```python
from build123d import *

# Parameters (mm, degrees)
BOSS_EXTRUDE1_DEPTH     = 28.8
CUT_EXTRUDE1_DEPTH      = 41.90409515
BOSS_EXTRUDE3_DEPTH     = 1
CUT_EXTRUDE2_DEPTH      = 4.7
BOSS_EXTRUDE2_START     = -0.8
BOSS_EXTRUDE2_OUTLINE_R = 2.3
BOSS_EXTRUDE2_DEPTH     = 0.8
SKETCH5_OUTSIDE_W       = 57.418
SKETCH5_OUTSIDE_H       = 48.718
CUT_EXTRUDE3_DEPTH      = 3.5
SKETCH6_OUTSIDE_W       = 57.418
SKETCH6_OUTSIDE_H       = 48.718
CUT_EXTRUDE4_DEPTH      = 2.5
SKETCH8_W               = 6.84
SKETCH8_H               = 4.95
BOSS_EXTRUDE4_DEPTH     = 25


# Read off the part's stored shape, not the designer's step: Boss-Extrude2
with BuildPart() as part:
    # Sketch1 → Boss-Extrude1 (new body)
    with BuildSketch(Plane(origin=(0, 0, 0), x_dir=(1, 0, 0), z_dir=(0, 1, 0))):
        with BuildLine():
            Line((-4, 13.05), (4, 13.05))
            ThreePointArc((4, 13.05), (8.213640499, 11.465985784), (11.656602829, 8.566006872))
            ThreePointArc((11.656602829, 8.566006872), (12.685480206, 7.779523995), (13.95, 7.5))
            Line((13.95, 7.5), (25.95, 7.5))
            Line((25.95, 7.5), (25.95, -7.5))
            Line((25.95, -7.5), (13.95, -7.5))
            ThreePointArc((13.95, -7.5), (12.685480206, -7.779523995), (11.656602829, -8.566006872))
            ThreePointArc((11.656602829, -8.566006872), (8.213640499, -11.465985784), (4, -13.05))
            Line((4, -13.05), (-4, -13.05))
            ThreePointArc((-4, -13.05), (-17.05, 0), (-4, 13.05))
        make_face()
    extrude(amount=-BOSS_EXTRUDE1_DEPTH)

    # Sketch2 → Cut-Extrude1 (cut, through all)
    with BuildSketch(Plane(origin=(0, 0, 0), x_dir=(1, 0, 0), z_dir=(0, 1, 0))):
        with BuildLine():
            Line((0, -9.05), (-4.7, -9.05))
            ThreePointArc((-4.7, -9.05), (-13.75, 0), (-4.7, 9.05))
            Line((-4.7, 9.05), (0, 9.05))
            ThreePointArc((0, 9.05), (9.05, 0), (0, -9.05))
        make_face()
    extrude(amount=-CUT_EXTRUDE1_DEPTH, mode=Mode.SUBTRACT)

    # Sketch7 → Boss-Extrude3 (add)
    with BuildSketch(Plane(origin=(0, 0, 0), x_dir=(1, 0, 0), z_dir=(0, 1, 0))):
        with BuildLine():
            Line((-4.7, 10.05), (0, 10.05))
            ThreePointArc((0, 10.05), (10.05, 0), (0, -10.05))
            Line((0, -10.05), (-4.7, -10.05))
            ThreePointArc((-4.7, -10.05), (-14.75, 0), (-4.7, 10.05))
        make_face()
    extrude(amount=-BOSS_EXTRUDE3_DEPTH)

    # Sketch3 → Cut-Extrude2 (cut)
    with BuildSketch(Plane(origin=(0, 0, 0), x_dir=(1, 0, 0), z_dir=(0, 1, 0))):
        with BuildLine():
            Line((25.95, 7.5), (18.35, 7.5))
            ThreePointArc((18.35, 7.5), (19.55, 0), (18.35, -7.5))
            Line((18.35, -7.5), (25.95, -7.5))
            Line((25.95, -7.5), (25.95, 7.5))
        make_face()
    extrude(amount=-CUT_EXTRUDE2_DEPTH, mode=Mode.SUBTRACT)

    # Boss-Extrude2 outline → Boss-Extrude2 (add)
    # profile 1 of 2: a face of its own
    with BuildSketch(Plane(origin=(0, -15.8, 0), x_dir=(1, 0, 0), z_dir=(0, 1, 0)).offset(BOSS_EXTRUDE2_START)):
        with BuildLine():
            Line((17.95, -13.1), (17.95, -12.5))
            Line((17.95, -12.5), (18.65, -12.5))
            Line((18.65, -12.5), (18.65, -7.5))
            Line((18.65, -7.5), (13.95, -7.5))
            ThreePointArc((13.95, -7.5), (12.685480206, -7.779523995), (11.656602829, -8.566006872))
            ThreePointArc((11.656602829, -8.566006872), (9.898058886, -10.29612198), (7.85, -11.671341923))
            Line((7.85, -11.671341923), (7.85, -12.335141167))
            ThreePointArc((7.85, -12.335141167), (7.996446609, -12.688694558), (8.35, -12.835141167))
            Line((8.35, -12.835141167), (9.85, -12.835141167))
            Line((9.85, -12.835141167), (9.85, -13.1))
            ThreePointArc((9.85, -13.1), (13.9, -17.15), (17.95, -13.1))
        make_face()
        with Locations((13.9, -13.1)):
            Circle(BOSS_EXTRUDE2_OUTLINE_R, mode=Mode.SUBTRACT)
    # profile 2 of 2: a face of its own
    with BuildSketch(Plane(origin=(0, -15.8, 0), x_dir=(1, 0, 0), z_dir=(0, 1, 0)).offset(BOSS_EXTRUDE2_START)):
        with BuildLine():
            Line((17.95, 12.5), (17.95, 13.1))
            ThreePointArc((17.95, 13.1), (13.9, 17.15), (9.85, 13.1))
            Line((9.85, 13.1), (9.85, 12.835141167))
            Line((9.85, 12.835141167), (8.35, 12.835141167))
            ThreePointArc((8.35, 12.835141167), (7.996446609, 12.688694558), (7.85, 12.335141167))
            Line((7.85, 12.335141167), (7.85, 11.671341923))
            ThreePointArc((7.85, 11.671341923), (9.898058886, 10.29612198), (11.656602829, 8.566006872))
            ThreePointArc((11.656602829, 8.566006872), (12.685480206, 7.779523995), (13.95, 7.5))
            Line((13.95, 7.5), (18.65, 7.5))
            Line((18.65, 7.5), (18.65, 12.5))
            Line((18.65, 12.5), (17.95, 12.5))
        make_face()
        with Locations((13.9, 13.1)):
            Circle(BOSS_EXTRUDE2_OUTLINE_R, mode=Mode.SUBTRACT)
    extrude(amount=BOSS_EXTRUDE2_DEPTH)

    # Sketch5 outside → Cut-Extrude3 (cut)
    # profile 1 of 2: a face of its own
    with BuildSketch(Plane.XZ.offset(28.8)):
        with Locations((4.45, 0)):
            Rectangle(SKETCH5_OUTSIDE_W, SKETCH5_OUTSIDE_H)
        with BuildLine():
            Line((-4.7, -11.05), (0, -11.05))
            ThreePointArc((0, -11.05), (11.05, 0), (0, 11.05))
            Line((0, 11.05), (-4.7, 11.05))
            ThreePointArc((-4.7, 11.05), (-15.75, 0), (-4.7, -11.05))
        make_face(mode=Mode.SUBTRACT)
    # profile 2 of 2: a face of its own
    with BuildSketch(Plane.XZ.offset(28.8)):
        with BuildLine():
            Line((-4.7, 9.05), (0, 9.05))
            ThreePointArc((0, 9.05), (9.05, 0), (0, -9.05))
            Line((0, -9.05), (-4.7, -9.05))
            ThreePointArc((-4.7, -9.05), (-13.75, 0), (-4.7, 9.05))
        make_face()
    extrude(amount=-CUT_EXTRUDE3_DEPTH, mode=Mode.SUBTRACT)

    # Sketch6 outside → Cut-Extrude4 (cut)
    with BuildSketch(Plane.XZ.offset(25.3)):
        with Locations((4.45, 0)):
            Rectangle(SKETCH6_OUTSIDE_W, SKETCH6_OUTSIDE_H)
        with BuildLine():
            Line((-0.915214063, 14.471830711), (-20.749472671, 14.471830711))
            Line((-20.749472671, 14.471830711), (-20.749472671, -14.500741391))
            Line((-20.749472671, -14.500741391), (0, -14.500741391))
            ThreePointArc((0, -14.500741391), (14.493511919, 0.457835289), (-0.915214063, 14.471830711))
        make_face(mode=Mode.SUBTRACT)
    extrude(amount=-CUT_EXTRUDE4_DEPTH, mode=Mode.SUBTRACT)

    # Sketch8 → Boss-Extrude4 (add)
    with BuildSketch(Plane(origin=(25.95, 0, 0), x_dir=(0, 0, -1), z_dir=(1, 0, 0))):
        with Locations((0, -19.505)):
            Rectangle(SKETCH8_W, SKETCH8_H)
        with Locations((0, -8.555)):
            Rectangle(SKETCH8_W, SKETCH8_H)
    extrude(amount=-BOSS_EXTRUDE4_DEPTH)


solid = part.part
```
Work out the finished part from the listing and answer in its coordinate system (mm). A direction names the side the tool comes from. Give positions to 0.01 mm unless a question says otherwise; leave off trailing zeros. Loops run counter-clockwise (first coordinate to the right, second up) from the corner with the lowest first, then second, coordinate; pieces in that order, holes last. Notation, with made-up numbers: (-36, 67.25) -> (-23, 67.25) arc R26 cw to (-23, 87.25) -> close; hole circle Ø3 at (27.5, 34.25). An arc over 180 degrees is marked (long way). One line per question, with ' | ' between items. Start each with the question number.
1) Section B-B, the plane z = 0 is taken. Determine the outline of the cut face in (x, y).
2) Determine the mould class of faces 1 (the face through (0.95, -19, 0)), 2 (the face through (0, -12, 13.05)), 3 (the face through (22, -4.7, 0)) for opening direction Z: +Z half, -Z half, draft (parallel to the pull), parting line (faces both ways), or undercut.
3) Section D-D, the plane x = 22 is taken. Determine the outline of the cut face in (y, z).
4) Straight lines are drawn through the part: L1, parallel to Z at x = 13.9, y = -16.3; L2, parallel to Z at x = 3.5, y = -8.25; L3, parallel to Y at x = 1.5, z = -1. For each, find the intervals that lie inside material, in ascending order.
5) Each of these flat-tipped pins is pushed along its axis until it touches: pin 1 (0.5 mm diameter, centred on y = -16, z = 13, fed in from +X); pin 2 (5 mm diameter, centred on x = -5.5, y = -4.5, fed in from -Z); pin 3 (6 mm diameter, centred on x = -10.5, y = -6, fed in from +Z). Where does it stop, or does it pass through?
6) For faces 4 (the face through (9.048, -14.705, -0.199)), 5 (the face through (16, -15.8, -11)), 6 (the face through (5, -21.98, 0)), 7 (the face through (12.702, -7.789, 7.772)), determine the directions among +Z, -Z, +X, -X, +Y, -Y from which every point of the face is accessible in a straight line to the end or side of a thin tool.
7) Section C-C, the plane y = -24.5 is taken. Determine the outline of the cut face in (x, z).
8) Section A-A, the plane y = -10 is taken. Determine the outline of the cut face in (x, z).
Resolved:
1) outline: (-17.05, -25.3) -> (-15.75, -25.3) -> (-15.75, -28.8) -> (-13.75, -28.8) -> (-13.75, -1) -> (9.05, -1) -> (9.05, -6.08) -> (0.95, -6.08) -> (0.95, -11.03) -> (9.05, -11.03) -> (9.05, -17.03) -> (0.95, -17.03) -> (0.95, -21.98) -> (9.05, -21.98) -> (9.05, -28.8) -> (11.05, -28.8) -> (11.05, -25.3) -> (14.5, -25.3) -> (14.5, -22.8) -> (25.95, -22.8) -> (25.95, -4.7) -> (19.55, -4.7) -> (19.55, 0) -> (-17.05, 0) -> close
2) face 1: undercut | face 2: +Z half | face 3: draft
3) outline: (-22.8, -7.5) -> (-4.7, -7.5) -> (-4.7, 7.5) -> (-22.8, 7.5) -> close
4) L1: -17.15 to -15.4, -10.8 to 10.8, 15.4 to 17.15 | L2: -13.05 to -8.35, -3.42 to 3.42, 8.35 to 13.05 | L3: -21.98 to -17.03, -11.03 to -6.08, -1 to 0
5) pin 1: x = 17.95 | pin 2: z = -13.05 | pin 3: z = 12.57
6) face 4: none | face 5: -Z, +X, +Y | face 6: -Y | face 7: +Z, +X, +Y
7) outline: (-4, -13.05) -> (4, -13.05) arc R13.29 ccw to (11.66, -8.57) arc R3 cw to (11.85, -8.36) arc R14.5 ccw to (11.85, 8.36) arc R3 cw to (11.66, 8.57) arc R13.29 ccw to (4, 13.05) -> (-4, 13.05) arc R13.05 ccw to start; hole (-4.7, -9.05) -> (0, -9.05) arc R9.05 ccw to (0, 9.05) -> (-4.7, 9.05) arc R9.05 ccw to start
8) outline: (-4, -13.05) -> (4, -13.05) arc R13.29 ccw to (11.66, -8.57) arc R3 cw to (13.95, -7.5) -> (25.95, -7.5) -> (25.95, 7.5) -> (13.95, 7.5) arc R3 cw to (11.66, 8.57) arc R13.29 ccw to (4, 13.05) -> (-4, 13.05) arc R13.05 ccw to start; hole (-4.7, -9.05) -> (0, -9.05) arc R9.05 ccw to (8.38, -3.42) -> (0.95, -3.42) -> (0.95, 3.42) -> (8.38, 3.42) arc R9.05 ccw to (0, 9.05) -> (-4.7, 9.05) arc R9.05 ccw to start
